Geometry check sheet. Reference: the model listing, model coordinates, mm. Give positions to 0.01 mm unless a question says otherwise; leave off trailing zeros. Order: outer loops, then holes, each group sorted by start corner. A loop starts at its lowest first (then second) coordinate and runs counter-clockwise, first axis right, second up. Notation, with made-up numbers: (42, -27.75) - (56, -27.75) arc R14 ccw to (56, -22.75) - close; hole circle Ø4 at (60.25, -35.5). An arc over 180 degrees is marked (long way). Put each result on its own line as item: value. Start each with the question number.
```python
from build123d import *

# Parameters (mm, degrees)
SKETCH_1_W          = 30
SKETCH_1_H          = 20
SKETCH_1_W_2        = 28
SKETCH_1_H_2        = 18
EXTRUDE_1_DEPTH     = 297.5
SKETCH_2_R          = 2
CUT_EXTRUDE_1_DEPTH = 70
CUT_EXTRUDE_2_DEPTH = 65
SKETCH_5_R          = 2
CUT_EXTRUDE_3_DEPTH = 35


with BuildPart() as part:
    # 草图1 → 凸台-拉伸1 (new, symmetric)
    with BuildSketch(Plane.XY):
        Rectangle(SKETCH_1_W, SKETCH_1_H)
        Rectangle(SKETCH_1_W_2, SKETCH_1_H_2, mode=Mode.SUBTRACT)
    extrude(amount=EXTRUDE_1_DEPTH, both=True)

    # 草图2 → 切除-拉伸1 (cut)
    with BuildSketch(Plane(origin=(0, 10, 0), x_dir=(1, 0, 0), z_dir=(0, 1, 0))):
        with Locations(Location((9, 79, 0), (0, 0, 270))):
            Circle(SKETCH_2_R)
        with Locations(Location((-9, 79, 0), (0, 0, 270))):
            Circle(SKETCH_2_R)
        with Locations(Location((-9, 61, 0), (0, 0, 270))):
            Circle(SKETCH_2_R)
        with Locations(Location((9, 61, 0), (0, 0, 270))):
            Circle(SKETCH_2_R)
    cut_extrude_1 = extrude(amount=-CUT_EXTRUDE_1_DEPTH, mode=Mode.SUBTRACT)

    # 镜向1: 切除-拉伸1 across plane
    add(cut_extrude_1.mirror(Plane.XY), mode=Mode.SUBTRACT)

    # 草图4 → 切除-拉伸2 (cut)
    with BuildSketch(Plane(origin=(15, 0, 0), x_dir=(0, 0, -1), z_dir=(1, 0, 0))):
        with BuildLine():
            Line((-79, 4), (-61, 4))
            ThreePointArc((-61, 4), (-57, 0), (-61, -4))
            Line((-61, -4), (-79, -4))
            ThreePointArc((-79, -4), (-83, 0), (-79, 4))
        make_face()
    cut_extrude_2 = extrude(amount=-CUT_EXTRUDE_2_DEPTH, mode=Mode.SUBTRACT)

    # 镜向2: 切除-拉伸2 across plane
    add(cut_extrude_2.mirror(Plane.XY), mode=Mode.SUBTRACT)

    # 草图5 → 切除-拉伸3 (cut, symmetric)
    with BuildSketch(Plane.XZ.offset(10)):
        with Locations(Location((0, -244, 0), (0, 0, 270))):
            Circle(SKETCH_5_R)
        with Locations(Location((0, -214, 0), (0, 0, 270))):
            Circle(SKETCH_5_R)
    cut_extrude_3 = extrude(amount=CUT_EXTRUDE_3_DEPTH, both=True, mode=Mode.SUBTRACT)

    # 镜向3: 切除-拉伸3 across plane
    add(cut_extrude_3.mirror(Plane.XY), mode=Mode.SUBTRACT)


solid = part.part
```
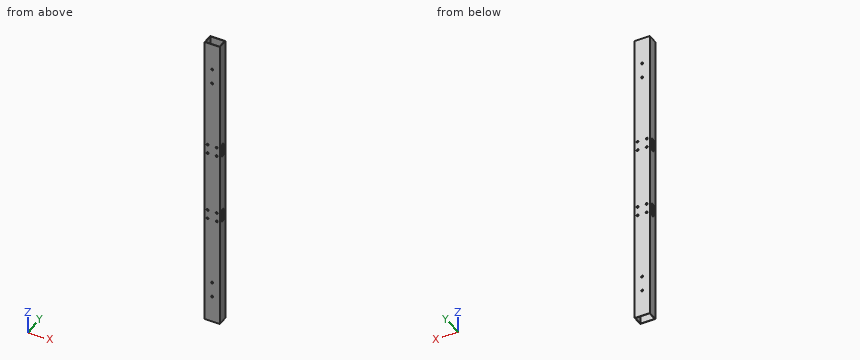
Item 1: Cross-section at A-A (z = 68). Enter the section's corners in (x, y).
Item 2: Cross-section at B-B (z = -182.5). Enter the section's corners in (x, y).
Item 3: Thickness scan on line 1 along X through (y, z) = (9.65, 61); line 2 along Y through (x, z) = (0.5, -57.5); line 3 along X through (y, z) = (7, 169). Record the ranges inside material, lowest first.
Recorded:
1. outline: (-15, -10) - (15, -10) - (15, -4) - (14, -4) - (14, -9) - (-14, -9) - (-14, -4) - (-15, -4) - close; (-15, 4) - (-14, 4) - (-14, 9) - (14, 9) - (14, 4) - (15, 4) - (15, 10) - (-15, 10) - close
2. outline: (-15, -10) - (15, -10) - (15, 10) - (-15, 10) - close; hole (-14, -9) - (14, -9) - (14, 9) - (-14, 9) - close
3. line 1: x = -15 to -11, -7 to 7, 11 to 15
3. line 2: y = -10 to -9, 9 to 10
3. line 3: x = -15 to -14, 14 to 15
